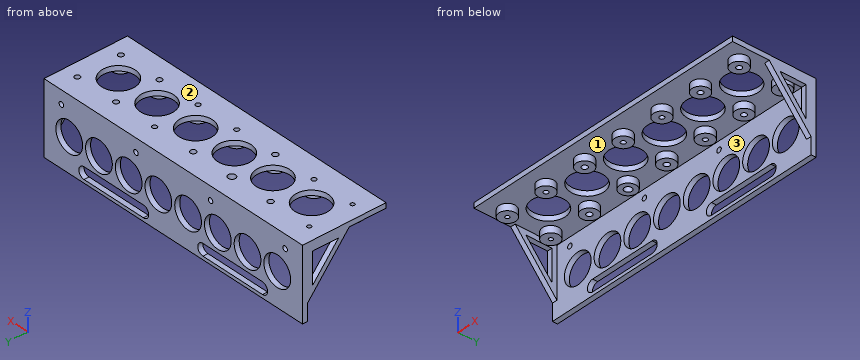
from build123d import *

# Parameters (mm, degrees)
SKETCH_W      = 174
SKETCH_H      = 50
SKETCH_R      = 1.2
SKETCH_R_2    = 1.7
SKETCH_R_3    = 1.4
SKETCH_R_4    = 2.2
SKETCH_R_5    = 1.6
SKETCH_R_6    = 10
PAD_DEPTH     = 3
SKETCH002_W   = 174
SKETCH002_H   = 40
SKETCH002_R   = 9
SKETCH002_R_2 = 1.5
PAD002_DEPTH  = 3
PAD003_DEPTH  = 3
PAD004_DEPTH  = 3
SKETCH001_R   = 5
SKETCH001_R_2 = 1.2
SKETCH001_R_3 = 1.7
SKETCH001_R_4 = 1.4
SKETCH001_R_5 = 2.2
SKETCH001_R_6 = 1.6
PAD001_DEPTH  = 4


with BuildPart() as pad:
    # Sketch → Pad (new body)
    with BuildSketch(Plane.XY):
        Rectangle(SKETCH_W, SKETCH_H)
        with Locations((-78, 13)):
            Circle(SKETCH_R, mode=Mode.SUBTRACT)
        with Locations((-78, -13)):
            Circle(SKETCH_R, mode=Mode.SUBTRACT)
        with Locations((-52, 13)):
            Circle(SKETCH_R_2, mode=Mode.SUBTRACT)
        with Locations((-52, -13)):
            Circle(SKETCH_R_3, mode=Mode.SUBTRACT)
        with Locations((-26, 13)):
            Circle(SKETCH_R_4, mode=Mode.SUBTRACT)
        with Locations((-26, -13)):
            Circle(SKETCH_R_2, mode=Mode.SUBTRACT)
        with Locations((0, 13)):
            Circle(SKETCH_R_2, mode=Mode.SUBTRACT)
        with Locations((0, -13)):
            Circle(SKETCH_R_3, mode=Mode.SUBTRACT)
        with Locations((26, 13)):
            Circle(SKETCH_R_3, mode=Mode.SUBTRACT)
        with Locations((26, -13)):
            Circle(SKETCH_R_3, mode=Mode.SUBTRACT)
        with Locations((52, 13)):
            Circle(SKETCH_R_5, mode=Mode.SUBTRACT)
        with Locations((52, -13)):
            Circle(SKETCH_R_5, mode=Mode.SUBTRACT)
        with Locations((78, 13)):
            Circle(SKETCH_R_5, mode=Mode.SUBTRACT)
        with Locations((78, -13)):
            Circle(SKETCH_R_5, mode=Mode.SUBTRACT)
        with Locations((-39, 0)):
            Circle(SKETCH_R_6, mode=Mode.SUBTRACT)
        with Locations((-13, 0)):
            Circle(SKETCH_R_6, mode=Mode.SUBTRACT)
        with Locations((13, 0)):
            Circle(SKETCH_R_6, mode=Mode.SUBTRACT)
        with Locations((39, 0)):
            Circle(SKETCH_R_6, mode=Mode.SUBTRACT)
        with Locations((65, 0)):
            Circle(SKETCH_R_6, mode=Mode.SUBTRACT)
        with Locations((-65, 0)):
            Circle(SKETCH_R_6, mode=Mode.SUBTRACT)
    extrude(amount=PAD_DEPTH)


with BuildPart() as pad002:
    # Sketch002 → Pad002 (new body)
    with BuildSketch(Plane(origin=(0, 25, -20), x_dir=(1, 0, 0), z_dir=(0, -1, 0))):
        Rectangle(SKETCH002_W, SKETCH002_H)
        with Locations((-70, 0)):
            Circle(SKETCH002_R, mode=Mode.SUBTRACT)
        with Locations((-50, 0)):
            Circle(SKETCH002_R, mode=Mode.SUBTRACT)
        with Locations((-30, 0)):
            Circle(SKETCH002_R, mode=Mode.SUBTRACT)
        with Locations((-10, 0)):
            Circle(SKETCH002_R, mode=Mode.SUBTRACT)
        with Locations((10, 0)):
            Circle(SKETCH002_R, mode=Mode.SUBTRACT)
        with Locations((30, 0)):
            Circle(SKETCH002_R, mode=Mode.SUBTRACT)
        with Locations((50, 0)):
            Circle(SKETCH002_R, mode=Mode.SUBTRACT)
        with Locations((70, 0)):
            Circle(SKETCH002_R, mode=Mode.SUBTRACT)
        with Locations((-75.3, 15)):
            Circle(SKETCH002_R_2, mode=Mode.SUBTRACT)
        with Locations((-25.1, 15)):
            Circle(SKETCH002_R_2, mode=Mode.SUBTRACT)
        with Locations((25.1, 15)):
            Circle(SKETCH002_R_2, mode=Mode.SUBTRACT)
        with Locations((75.3, 15)):
            Circle(SKETCH002_R_2, mode=Mode.SUBTRACT)
        with BuildLine():
            ThreePointArc((-60, -11), (-63.5, -14.5), (-60, -18))
            Line((-60, -18), (-20, -18))
            ThreePointArc((-20, -18), (-16.5, -14.5), (-19.999999, -11))
            Line((-60, -11), (-19.999999, -11))
        make_face(mode=Mode.SUBTRACT)
        with BuildLine():
            ThreePointArc((19.999985, -11), (16.5, -14.500007), (19.999999, -18))
            Line((19.999999, -18), (60.000001, -18))
            ThreePointArc((60.000001, -18), (63.5, -14.499993), (59.999987, -11))
            Line((19.999985, -11), (59.999987, -11))
        make_face(mode=Mode.SUBTRACT)
    extrude(amount=PAD002_DEPTH)


with BuildPart() as pad003:
    # Sketch003 → Pad003 (new body)
    with BuildSketch(Plane(origin=(-87, 22, 0), x_dir=(0, 1, 0), z_dir=(1, 0, 0))):
        Polygon((-25, 0), (0, 0), (0, -30), align=None)
        Polygon((-18.594875, -3), (-3, -3), (-3, -21.71385), align=None, mode=Mode.SUBTRACT)
    extrude(amount=PAD003_DEPTH)


with BuildPart() as pad004:
    # Sketch004 → Pad004 (new body)
    with BuildSketch(Plane(origin=(84, 22, 0), x_dir=(0, 1, 0), z_dir=(1, 0, 0))):
        Polygon((-25, 0), (0, 0), (0, -30), align=None)
        Polygon((-18.594875, -3), (-3, -3), (-3, -21.71385), align=None, mode=Mode.SUBTRACT)
    extrude(amount=PAD004_DEPTH)


with BuildPart() as fusion:
    # Sketch001 → Pad001 (new body)
    with BuildSketch(Plane.XY.offset(-4)):
        with Locations((-78, 13)):
            Circle(SKETCH001_R)
        with Locations((-78, 13)):
            Circle(SKETCH001_R_2, mode=Mode.SUBTRACT)
        with Locations((-78, -13)):
            Circle(SKETCH001_R)
        with Locations((-78, -13)):
            Circle(SKETCH001_R_2, mode=Mode.SUBTRACT)
        with Locations((-52, 13)):
            Circle(SKETCH001_R)
        with Locations((-52, 13)):
            Circle(SKETCH001_R_3, mode=Mode.SUBTRACT)
        with Locations((-52, -13)):
            Circle(SKETCH001_R)
        with Locations((-52, -13)):
            Circle(SKETCH001_R_4, mode=Mode.SUBTRACT)
        with Locations((-26, 13)):
            Circle(SKETCH001_R)
        with Locations((-26, 13)):
            Circle(SKETCH001_R_5, mode=Mode.SUBTRACT)
        with Locations((-26, -13)):
            Circle(SKETCH001_R)
        with Locations((-26, -13)):
            Circle(SKETCH001_R_3, mode=Mode.SUBTRACT)
        with Locations((0, 13)):
            Circle(SKETCH001_R)
        with Locations((0, 13)):
            Circle(SKETCH001_R_3, mode=Mode.SUBTRACT)
        with Locations((0, -13)):
            Circle(SKETCH001_R)
        with Locations((0, -13)):
            Circle(SKETCH001_R_4, mode=Mode.SUBTRACT)
        with Locations((26, 13)):
            Circle(SKETCH001_R)
        with Locations((26, 13)):
            Circle(SKETCH001_R_4, mode=Mode.SUBTRACT)
        with Locations((26, -13)):
            Circle(SKETCH001_R)
        with Locations((26, -13)):
            Circle(SKETCH001_R_4, mode=Mode.SUBTRACT)
        with Locations((52, 13)):
            Circle(SKETCH001_R)
        with Locations((52, 13)):
            Circle(SKETCH001_R_6, mode=Mode.SUBTRACT)
        with Locations((52, -13)):
            Circle(SKETCH001_R)
        with Locations((52, -13)):
            Circle(SKETCH001_R_6, mode=Mode.SUBTRACT)
        with Locations((78, 13)):
            Circle(SKETCH001_R)
        with Locations((78, 13)):
            Circle(SKETCH001_R_6, mode=Mode.SUBTRACT)
        with Locations((78, -13)):
            Circle(SKETCH001_R)
        with Locations((78, -13)):
            Circle(SKETCH001_R_6, mode=Mode.SUBTRACT)
    extrude(amount=PAD001_DEPTH)

    # Fusion: union Pad, Pad002, Pad003, Pad004
    add(pad.part)
    add(pad002.part)
    add(pad003.part)
    add(pad004.part)


solid = fusion.part
For this review, take the finished solid that the model builds, in its own axes (mm). Face numbers are marked on the shaded views. Round coordinates to 2 decimals unless told otherwise and drop trailing zeros. Loops run counter-clockwise (first coordinate to the right, second up) from the corner with the lowest first, then second, coordinate; pieces in that order, holes last. Notation, with made-up numbers: (24.25, 54.5) - (41.25, 54.5) arc R25 ccw to (41.25, 79.5) - close; hole circle Ø3 at (39, 89). An arc over 180 degrees is marked (long way). Put each result on its own line as item: value. Start each with the question number.
1. Mouldability with a two-part tool opening along X and no side actions: class the marked faces 1, 2 and 3 as +X half, -X half, draft (parallel to the pull), parting line (faces both ways), or undercut.
2. Insertion check: P1, Ø4, axis at x = 0, y = 13, coming from the -Z side; P2, Ø5, axis at x = -25.1, z = -5, coming from the -Y side; P3, Ø23.5, axis at x = -50, z = -20, coming from the -Y side. Each pin has a flat end and moves straight along its axis. Give the tip position at first contact, or say it passes through.
3. Consider section B-B on z = -8. State the section outline as (x, y) points.
4. For probe 1 along Y at (x, z) = (-52, -2); probe 2 along Y at (x, z) = (78, 1); probe 3 along Z at (x, y) = (69.5, 23), list the stretches that pass through material, from the lowest coordinate up. Write a range as [from, to].
5. Consider section D-D on x = -36.5. State the section outline as (y, z) points, plus the area to 3 significant figures.
6. Consider section C-C on x = -12. State the section outline as (y, z) points.
7. Consider section A-A on y = -6. State the section outline as (x, z) points.
Result sheet:
1. face 1: undercut
1. face 2: draft
1. face 3: undercut
2. P1: z = -4
2. P2: y = -18
2. P3: y = 22
3. outline: (-87, 3.67) - (-84, 3.67) - (-84, 7.57) - (-87, 7.57) - close; (-87, 19) - (-84, 19) - (-84, 22) - (84, 22) - (84, 19) - (87, 19) - (87, 25) - (-87, 25) - close; (84, 3.67) - (87, 3.67) - (87, 7.57) - (84, 7.57) - close
4. probe 1: [-18, -14.4], [-11.6, -8], [8, 11.3], [14.7, 18], [22, 25]
4. probe 2: [-25, -14.6], [-11.4, 11.4], [14.6, 25]
4. probe 3: [-40, -28.99], [-11.01, 3]
5. outline: (-25, 0) - (-9.68, 0) - (-9.68, 3) - (-25, 3) - close; (9.68, 0) - (22, 0) - (22, -13.78) - (25, -13.78) - (25, 3) - (9.68, 3) - close; (22, -40) - (25, -40) - (25, -38) - (22, -38) - close; (22, -31) - (25, -31) - (25, -26.22) - (22, -26.22) - close
5. area: 154 mm^2
6. outline: (-25, 0) - (-9.95, 0) - (-9.95, 3) - (-25, 3) - close; (9.95, 0) - (22, 0) - (22, -11.23) - (25, -11.23) - (25, 3) - (9.95, 3) - close; (22, -40) - (25, -40) - (25, -28.77) - (22, -28.77) - close
7. outline: (-87, 0) - (-73, 0) - (-73, 3) - (-87, 3) - close; (-57, 0) - (-47, 0) - (-47, 3) - (-57, 3) - close; (-31, 0) - (-21, 0) - (-21, 3) - (-31, 3) - close; (-5, 0) - (5, 0) - (5, 3) - (-5, 3) - close; (21, 0) - (31, 0) - (31, 3) - (21, 3) - close; (47, 0) - (57, 0) - (57, 3) - (47, 3) - close; (73, 0) - (87, 0) - (87, 3) - (73, 3) - close
